For this review, take the finished solid that the model builds, in its own axes (mm). A direction names the side the tool comes from. Coordinates: 2 decimals unless noted, no trailing zeros. Loops run counter-clockwise (first coordinate to the right, second up) from the corner with the lowest first, then second, coordinate; pieces in that order, holes last. Notation, with made-up numbers: M -39,11 L -24,11 A9 ccw -24,16 Z; hole C 87.25,56 d2. An arc over 180 degrees is marked long. Write item = value, one per line.
from build123d import *

# Parameters (mm, degrees)
SKETCH2_R               = 4
SKETCH2_R_2             = 3
BOSS_EXTRUDE1_DEPTH     = 10
CUT_EXTRUDE1_DEPTH      = 43.801869118
CUT_EXTRUDE1_DEPTH_BACK = 43.801869118
SKETCH3_R               = 1.5
SKETCH3_R_2             = 2
SKETCH4_W               = 13
SKETCH4_H               = 38
CUT_EXTRUDE2_DEPTH      = 10


with BuildPart() as part:
    # Sketch1 → Revolve1 (revolve)
    with BuildSketch(Plane.XY, mode=Mode.PRIVATE) as revolve1_sk:
        Polygon((3, 0), (4, 0), (4, 14), (18, 14), (18, 22), (0, 22), (0, 13), (3, 13), align=None)
    revolve(revolve1_sk.sketch.rotate(Axis((0, 0, 0), (0, 1, 0)), 90), axis=Axis((0, 0, 0), (0, 1, 0)))

    # Sketch2 → Boss-Extrude1 (add)
    with BuildSketch(Plane(origin=(0, 22, 0), x_dir=(1, 0, 0), z_dir=(0, 1, 0))):
        with Locations(Location((0, 0, 0), (0, 0, 90))):
            Circle(SKETCH2_R)
        with Locations(Location((0, 0, 0), (0, 0, 90))):
            Circle(SKETCH2_R_2, mode=Mode.SUBTRACT)
    extrude(amount=BOSS_EXTRUDE1_DEPTH)

    # Sketch3 → Cut-Extrude1 (cut, two sides: drawn at the far end of the back side and taken through both)
    with BuildSketch(Plane(origin=(0, 0, -4), x_dir=(-1, 0, 0), z_dir=(0, 0, -1)).offset(-CUT_EXTRUDE1_DEPTH_BACK)):
        with Locations((0, 5)):
            Circle(SKETCH3_R)
        with Locations((0, 27)):
            Circle(SKETCH3_R)
        with Locations((0, 18)):
            Circle(SKETCH3_R_2)
    extrude(amount=CUT_EXTRUDE1_DEPTH + CUT_EXTRUDE1_DEPTH_BACK, mode=Mode.SUBTRACT)

    # Sketch4 → Cut-Extrude2 (cut)
    with BuildSketch(Plane(origin=(0, 22, 0), x_dir=(1, 0, 0), z_dir=(0, 1, 0))):
        with Locations((-16.5, 0)):
            Rectangle(SKETCH4_W, SKETCH4_H)
        with Locations((16.5, 0)):
            Rectangle(SKETCH4_W, SKETCH4_H)
    extrude(amount=-CUT_EXTRUDE2_DEPTH, mode=Mode.SUBTRACT)


solid = part.part
Q1. For pin 1 Ø5 at (x, y) = (0, 18) entering from -Z; pin 2 Ø4 at (x, y) = (0, 5) entering from +Z; pin 3 Ø3 at (x, y) = (4, 18) entering from +Z; pin 4 Ø5 at (x, z) = (0, 0) entering from -Y, all flat-tipped, find the tip position at first contact; note any pin that passes through.
Solved:
pin_1 = -18
pin_2 = 4
pin_3 = 17.83
pin_4 = 13
Q2. Draft analysis for pull direction Z (two halves, no side actions). For faces 4 (the face through (0, 22, 0)), 5 (the face through (-10, 18, 0)), 6 (the face through (-2.496, 18.056, 17.826)), state which applies: +Z half, -Z half, draft (parallel to the pull), parting line (faces both ways), or undercut.
Solved:
face_4 = undercut
face_5 = draft
face_6 = +Z half
Q3. Machinability: for faces 1 (the face through (1.532, 7.098, -3.695)), 2 (the face through (1.8, 26.9, 2.4)), 3 (the face through (-3, 0, 1)), which of the approach directions +Z, -Z, +X, -X, +Y, -Y give a long, thin tool a straight path to every point of the face, cutting with its end or side? Answer none if there is none.
Solved:
face_1 = -Y
face_2 = +Y
face_3 = +Z, -Z, +X, -X, -Y
Q4. Add section B-B (y = 27). Write out the cut boundary in (x, z).
Solved:
outline = M -1.5,-3.71 L -1.5,-2.6 A3 cw -1.5,2.6 L -1.5,3.71 A4 ccw Z; M 1.5,-3.71 A4 ccw 1.5,3.71 L 1.5,2.6 A3 cw 1.5,-2.6 Z
Q5. For line 1 along Y through (x, z) = (0, 3.2); line 2 along X through (y, z) = (29, 0); line 3 along Y through (x, z) = (0, 2.95), list the stretches that pass through material, from the lowest coordinate up.
Solved:
line_1 = 0 to 3.5, 6.5 to 16, 20 to 25.5, 28.5 to 32
line_2 = -4 to -3, 3 to 4
line_3 = 13 to 16, 20 to 22
Q6. Add section C-C (x = 0). State how many separate pieces and enclosed holes the cut face has, and give its area (3 significant figures).
Solved:
separate_pieces = 6
enclosed_holes = 0
area = 186 mm²
Q7. Add section A-A (z = 7). Write out the cut boundary in (x, y), and give its area (3 significant figures).
Solved:
outline = M -10,14 L 10,14 L 10,22 L -10,22 Z; hole C 0,18 d4
area = 147 mm²
Q8. Add section D-D (y = 4). Write out the cut boundary in (x, z), and give its area (3 significant figures).
Solved:
outline = M -1.12,-3.84 L -1.12,-2.78 A3 cw -1.12,2.78 L -1.12,3.84 A4 ccw Z; M 1.12,-3.84 A4 ccw 1.12,3.84 L 1.12,2.78 A3 cw 1.12,-2.78 Z
area = 17.4 mm²
